from build123d import *

# Parameters (mm, degrees)
SKETCH1_W           = 54
SKETCH1_H           = 45
BOSS_EXTRUDE1_DEPTH = 5
SKETCH3_W           = 5
SKETCH3_H           = 15
SKETCH3_W_2         = 15
SKETCH3_H_2         = 5
BOSS_EXTRUDE2_DEPTH = 5
SKETCH4_R           = 2
CUT_EXTRUDE1_DEPTH  = 5
SKETCH5_R           = 4
SKETCH5_R_2         = 2
BOSS_EXTRUDE3_DEPTH = 5


with BuildPart() as part:
    # Sketch1 → Boss-Extrude1 (new body)
    with BuildSketch(Plane.XY):
        Rectangle(SKETCH1_W, SKETCH1_H)
    extrude(amount=BOSS_EXTRUDE1_DEPTH)

    # Sketch3 → Boss-Extrude2 (add)
    with BuildSketch(Plane.XY.offset(5)):
        with Locations((29.5, 0)):
            Rectangle(SKETCH3_W, SKETCH3_H)
        with Locations((0, 25)):
            Rectangle(SKETCH3_W_2, SKETCH3_H_2)
    extrude(amount=-BOSS_EXTRUDE2_DEPTH)

    # Sketch4 → Cut-Extrude1 (cut)
    with BuildSketch(Plane.XY.offset(5)):
        with Locations((29.5, 0)):
            Circle(SKETCH4_R)
    extrude(amount=-CUT_EXTRUDE1_DEPTH, mode=Mode.SUBTRACT)

    # Sketch5 → Boss-Extrude3 (add)
    with BuildSketch(Plane.XY.offset(5)):
        with Locations((29.5, 0)):
            Circle(SKETCH5_R)
        with Locations((29.5, 0)):
            Circle(SKETCH5_R_2, mode=Mode.SUBTRACT)
    extrude(amount=-BOSS_EXTRUDE3_DEPTH)


solid = part.part
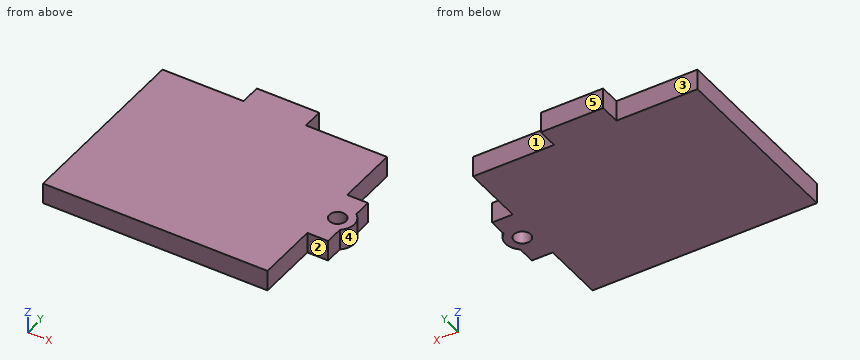
Verification items for the finished model (mm, model axes). Face numbers are marked on the shaded views. A direction names the side the tool comes from. Round coordinates to 2 decimals unless told otherwise and drop trailing zeros. Write each loop counter-clockwise with the first axis right and the second up, starting at its lowest first coordinate (ties: lowest second). Pieces come first, ordered by that corner, then holes.
(1) Depth check by flat-ended pin: pin 1 Ø1 at (x, y) = (13.5, 11.5) entering from -Z; pin 2 Ø2.5 at (x, y) = (29.5, 0) entering from +Z; pin 3 Ø1.5 at (x, z) = (29, 3) entering from -Y; pin 4 Ø1.5 at (y, z) = (12, 2) entering from +X. Enter the tip coordinate at first touch or a pass-through.
Returned:
pin 1: stops at z = 0
pin 2: passes through
pin 3: stops at y = -7.5
pin 4: stops at x = 27
(2) Section check C-C (x = 29.5). Enter the section's corners in (y, z), plus the area to 3 significant figures.
Returned:
outline: (-7.5, 0) - (-2, 0) - (-2, 5) - (-7.5, 5) - close; (2, 0) - (7.5, 0) - (7.5, 5) - (2, 5) - close
area: 55.0 mm2
(3) Access from +Z, -Z, +X, -X, +Y, -Y to the whole of each face (thin tool, end or side, straight path). Record for the marked faces 1, 2 and 3.
Returned:
face 1: +Z, -Z, +X, +Y
face 2: +Z, -Z, +X, -Y
face 3: +Z, -Z, -X, +Y
(4) Section check A-A (y = 0). Enter the section's corners in (x, z).
Returned:
outline: (-27, 0) - (27.5, 0) - (27.5, 5) - (-27, 5) - close; (31.5, 0) - (33.5, 0) - (33.5, 5) - (31.5, 5) - close
(5) Material ranges on line 1 (Y direction, x = 29.5, z = 3.95); line 2 (Y direction, x = 13, z = 1.95); line 3 (X direction, y = 15.5, z = 0.7), recorded low to high.
Returned:
line 1: y = -7.5 to -2, 2 to 7.5
line 2: y = -22.5 to 22.5
line 3: x = -27 to 27
(6) Section check D-D (x = 20). Enter the section's corners in (y, z).
Returned:
outline: (-22.5, 0) - (22.5, 0) - (22.5, 5) - (-22.5, 5) - close
(7) Section check B-B (z = 3.2). Enter the section's corners in (x, y).
Returned:
outline: (-27, -22.5) - (27, -22.5) - (27, -7.5) - (32, -7.5) - (32, -3.12) arc R4 ccw to (32, 3.12) - (32, 7.5) - (27, 7.5) - (27, 22.5) - (7.5, 22.5) - (7.5, 27.5) - (-7.5, 27.5) - (-7.5, 22.5) - (-27, 22.5) - close; hole circle Ø4 at (29.5, 0)
(8) Mould release check, pull along X, two halves, no side actions. Record for the marked faces 4 and 5: pulls with the +X half, pulls with the -X half, needs draft (parallel to the pull), parting line crosses it, or undercut.
Returned:
face 4: pulls with the +X half
face 5: needs draft
